Design review of the part built by this model. Coordinates are the model's own, in mm. Face numbers are marked on the shaded views. A direction names the side the tool comes from. Give positions to 0.01 mm unless a question says otherwise; leave off trailing zeros. Loops run counter-clockwise (first coordinate to the right, second up) from the corner with the lowest first, then second, coordinate; pieces in that order, holes last. Notation, with made-up numbers: M 14,14 L 61,14 A21 ccw 61,29 Z; hole C 36.5,79 d5. An arc over 180 degrees is marked long. Use a Markdown table: item, result. Add a question column.
(1) Draft analysis for pull direction X (two halves, no side actions). For the marked faces 3, 4 and 5, state which applies: pulls with the +X half, pulls with the -X half, needs draft (parallel to the pull), parting line crosses it, or undercut.
(2) For probe 1 along X at (y, z) = (-62, 72.5); probe 2 along Y at (x, z) = (95.5, 78); probe 3 along Z at (x, y) = (0, -99), list the stretches that pass through material, from the lowest coordinate up.
(3) Add section D-D, the plane x = 0. Give the boundary of the cut face in (y, z), then the cut area to 3 significant figures.
(4) Add section C-C, the plane z = 11.5. Give the boundary of the cut face in (x, y).
(5) For the marked faces 1 and 2, list the 3-axis set-ups (+Z, -Z, +X, -X, +Y, -Y) from which the entire face can be reached by the end or side of a thin tool; tool diameter is ignored.
(6) Insertion check: pin 1 Ø0.8 at (x, z) = (-111, 13.5) entering from -Y; pin 2 Ø3 at (y, z) = (57.5, 114.5) entering from +X; pin 3 Ø1.1 at (x, z) = (111, 90) entering from +Y. Each pin has a flat end and moves straight along its axis. Give the tip position at first contact, or say it passes through.
(7) Add section A-A, the plane x = -51. Give the boundary of the cut face in (y, z).
(8) Add section B-B, the plane y = -18. Give the boundary of the cut face in (x, z).
```python
from build123d import *

# Parameters (mm, degrees)
F0_W     = 223
F0_H     = 201
F1_DEPTH = 160
F2_W     = 221
F2_H     = 197
F3_DEPTH = 160
F4_W     = 150
F4_H     = 20
F5_DEPTH = 25
F6_W     = 150
F6_H     = 20
F7_DEPTH = 25
F8_R     = 10
F9_DEPTH = 25
F10_R    = 5


with BuildPart() as f1:
    # F0 (on Top) → F1 (new body)
    with BuildSketch(Plane.XY):
        Rectangle(F0_W, F0_H)
    extrude(amount=F1_DEPTH)

    # F2 (on face) → F3 (cut)
    with BuildSketch(Plane.XY.offset(160)):
        Rectangle(F2_W, F2_H)
    extrude(amount=-F3_DEPTH, mode=Mode.SUBTRACT)

    # F4 (on face) → F5 (cut)
    with BuildSketch(Plane.YZ.offset(111.5)):
        with Locations((0, 120)):
            Rectangle(F4_W, F4_H)
        with Locations((0, 90)):
            Rectangle(F4_W, F4_H)
    extrude(amount=-F5_DEPTH, mode=Mode.SUBTRACT)

    # F6 (on face) → F7 (cut)
    with BuildSketch(Plane(origin=(-111.5, 0, 0), x_dir=(0, -1, 0), z_dir=(-1, 0, 0))):
        with Locations((0, 15)):
            Rectangle(F6_W, F6_H)
    extrude(amount=-F7_DEPTH, mode=Mode.SUBTRACT)

    # F8 (on face) → F9 (cut)
    with BuildSketch(Plane.XZ.offset(100.5)):
        with Locations((0, 34.113634)):
            Circle(F8_R)
    extrude(amount=-F9_DEPTH, mode=Mode.SUBTRACT)

    # F10
    f10_edges = [f1.edges().sort_by_distance(p)[0] for p in [
        (-110.5, -98.5, 80),
        (-111.5, -100.5, 80),
        (-111.5, 100.5, 80),
        (-110.5, 98.5, 80),
        (110.5, 98.5, 80),
        (110.5, -98.5, 80),
        (111.5, 100.5, 80),
        (111.5, -100.5, 80),
    ]]
    fillet(f10_edges, radius=F10_R)


solid = f1.part
```
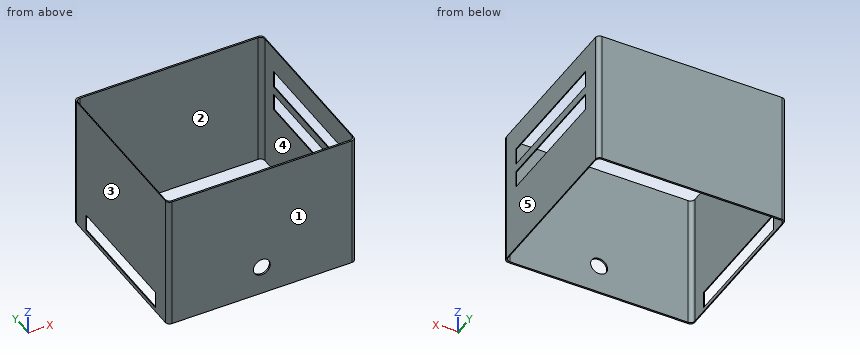
Established:
| question | item | result |
|---|---|---|
| 1 | face 3 | pulls with the -X half |
| 1 | face 4 | undercut |
| 1 | face 5 | pulls with the +X half |
| 2 | probe 1 | -111.5 to -110.5, 110.5 to 111.5 |
| 2 | probe 2 | -100.5 to -98.5, 98.5 to 100.5 |
| 2 | probe 3 | 0 to 24.11, 44.11 to 160 |
| 3 | outline | M -100.5,0 L -98.5,0 L -98.5,24.11 L -100.5,24.11 Z; M -100.5,44.11 L -98.5,44.11 L -98.5,160 L -100.5,160 Z; M 98.5,0 L 100.5,0 L 100.5,160 L 98.5,160 Z |
| 3 | area | 600 mm^2 |
| 4 | outline | M -111.5,-95.5 A5 ccw -106.5,-100.5 L 106.5,-100.5 A5 ccw 111.5,-95.5 L 111.5,95.5 A5 ccw 106.5,100.5 L -106.5,100.5 A5 ccw -111.5,95.5 L -111.5,75 L -110.5,75 L -110.5,93.5 A5 cw -105.5,98.5 L 105.5,98.5 A5 cw 110.5,93.5 L 110.5,-93.5 A5 cw 105.5,-98.5 L -105.5,-98.5 A5 cw -110.5,-93.5 L -110.5,-75 L -111.5,-75 Z |
| 5 | face 1 | +Z, -Z, +X, -X, -Y |
| 5 | face 2 | +Z, -Z |
| 6 | pin 1 | y = -98.36 |
| 6 | pin 2 | x = -110.5 |
| 6 | pin 3 | y = 98.57 |
| 7 | outline | M -100.5,0 L -98.5,0 L -98.5,160 L -100.5,160 Z; M 98.5,0 L 100.5,0 L 100.5,160 L 98.5,160 Z |
| 8 | outline | M -111.5,0 L -110.5,0 L -110.5,5 L -111.5,5 Z; M -111.5,25 L -110.5,25 L -110.5,160 L -111.5,160 Z; M 110.5,0 L 111.5,0 L 111.5,80 L 110.5,80 Z; M 110.5,100 L 111.5,100 L 111.5,110 L 110.5,110 Z; M 110.5,130 L 111.5,130 L 111.5,160 L 110.5,160 Z |
